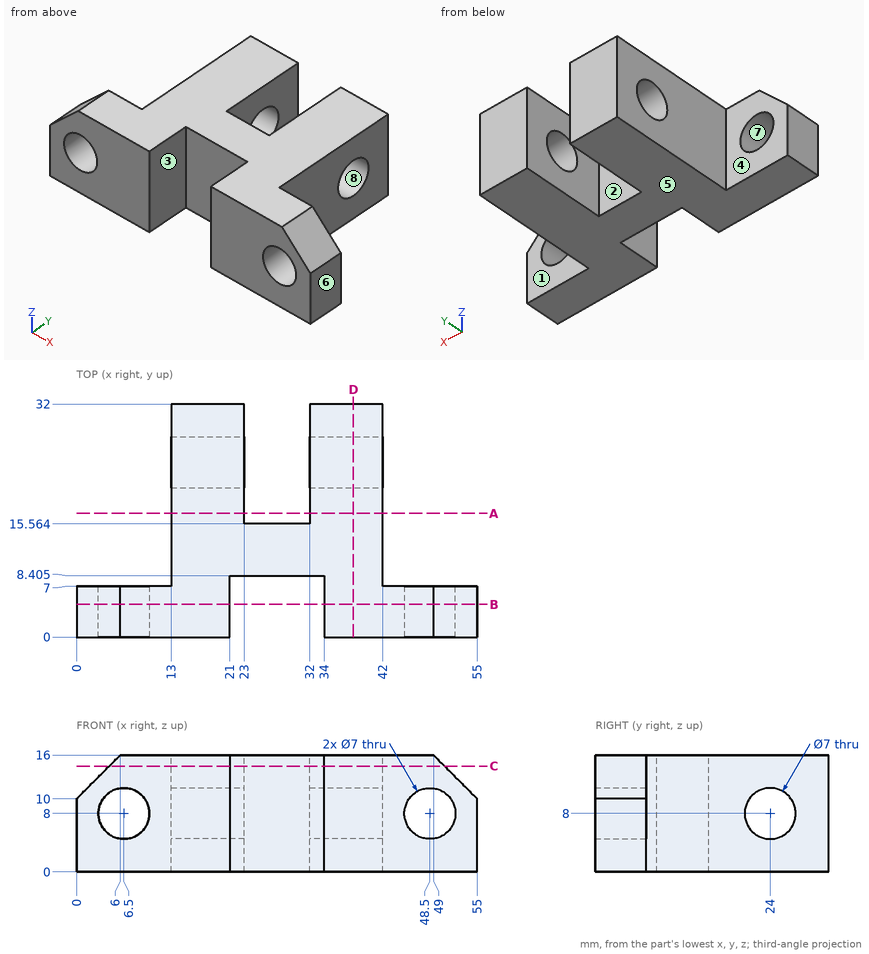
Drawing for the job (mm, zero at the part's lowest x, y, z). A direction names the side the tool comes from. Round coordinates to 2 decimals unless told otherwise and drop trailing zeros. Order: outer loops, then holes, each group sorted by start corner. A loop starts at its lowest first (then second) coordinate and runs counter-clockwise, first axis right, second up. Notation, with made-up numbers: M 38,9 L 69,9 A11 cw 69,20 Z; hole C 48.5,48 d9. An arc over 180 degrees is marked long. Use one line per item in the form item = value.
Q1. Which spindle directions (+Z, -Z, +X, -X, +Y, -Y) get a long thin tool onto all of the face, cutting with end or side? Do the marked faces 1, 2, 3 and 4. Say none if no direction does.
Recorded:
face_1 = +Z, -Z, +X, +Y
face_2 = +Z, -Z, +Y
face_3 = +Z, -Z, -Y
face_4 = +Z, -Z, -X, +Y
Q2. Saw through at C-C on z = 14.5. Give the cut face in (x, y) (1 decimal), then the cut area to 3 significant figures.
Recorded:
outline = M 4.5,0 L 21,0 L 21,8.4 L 34,8.4 L 34,0 L 50.5,0 L 50.5,7 L 42,7 L 42,32 L 32,32 L 32,15.6 L 23,15.6 L 23,32 L 13,32 L 13,7 L 4.5,7 Z
area = 790 mm^2
Q3. Two-plate mould, pull along Z, no slides. Class the marked faces 5, 6, 7 and 8: +Z half, -Z half, draft (parallel to the pull), parting line (faces both ways), or undercut.
Recorded:
face_5 = -Z half
face_6 = draft
face_7 = undercut
face_8 = undercut
Q4. Saw through at D-D on x = 38. Give the cut face in (y, z).
Recorded:
outline = M 0,0 L 32,0 L 32,16 L 0,16 Z; hole C 24,8 d7
Q5. Flat gauge pins, fed straight in: P1, Ø5.5, axis at y = 24, z = 8, coming from the +X side; P2, Ø5, axis at y = 16, z = 12, coming from the +X side; P3, Ø4, axis at x = 27, z = 5, coming from the -Y side (1 decimal); P4, Ø8, axis at y = 13.5, z = 9.5, coming from the -X side. Where does each tip first touch, or does it go through?
Recorded:
P1 = through
P2 = 42
P3 = 8.4
P4 = 13
Q6. Saw through at A-A on y = 17. Give the cut face in (x, z).
Recorded:
outline = M 13,0 L 23,0 L 23,16 L 13,16 Z; M 32,0 L 42,0 L 42,16 L 32,16 Z
Q7. Probe L1, parallel to X at y = 19, z = 14.75; L2, parallel to Z at x = 48.5, y = 5.5; L3, parallel to Y at x = 37.5, z = 8. List the from-to ranges inside material, lowest first.
Recorded:
L1 = 13 to 23, 32 to 42
L2 = 0 to 4.5, 11.5 to 16
L3 = 0 to 20.5, 27.5 to 32
Q8. Saw through at B-B on y = 4.5. Give the cut face in (x, z).
Recorded:
outline = M 0,0 L 21,0 L 21,16 L 6,16 L 0,10 Z; M 34,0 L 55,0 L 55,10 L 49,16 L 34,16 Z; hole C 6.5,8 d7; hole C 48.5,8 d7
